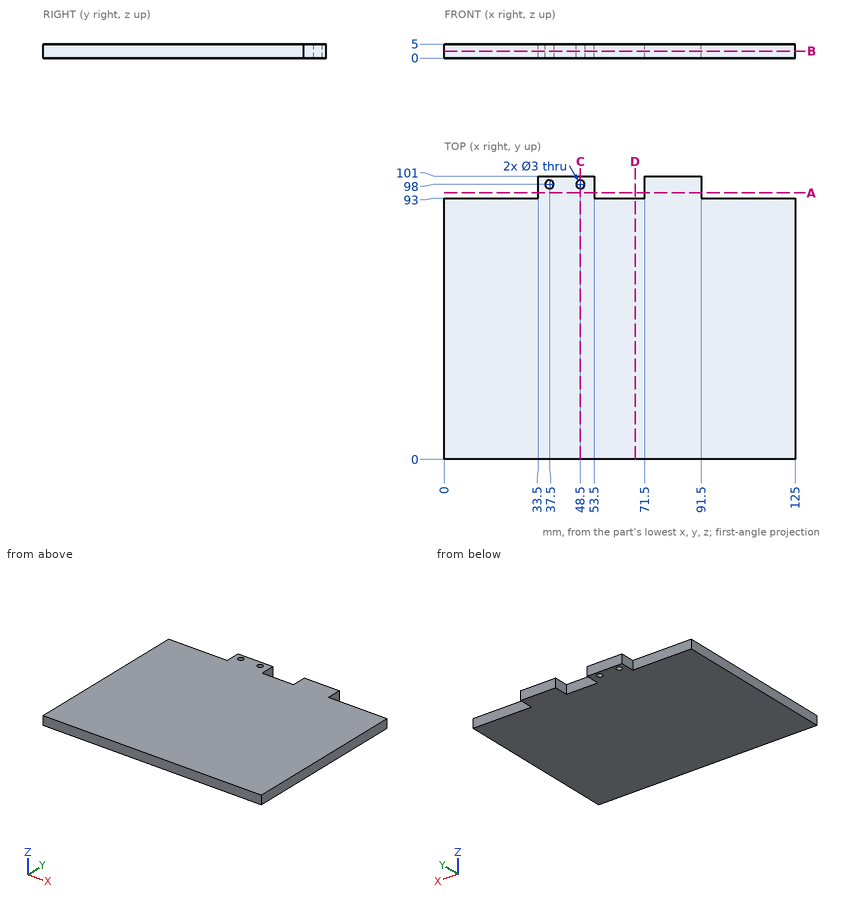
Could you check a few things on this drawing? It's one solid part, dimensions in mm from its lowest x, y, z. Give positions to 0.01 mm unless a question says otherwise; leave off trailing zeros. Order: outer loops, then holes, each group sorted by start corner. A loop starts at its lowest first (then second) coordinate and runs counter-clockwise, first axis right, second up. Notation, with made-up numbers: (49, -29) - (74, -29) arc R18 ccw to (74, 5) - close; hole circle Ø11 at (-20, 72). An arc over 180 degrees is marked (long way). One line per item, written item: value. Start each with the question number.
1. If I drill on probe 1 along X at (y, z) = (98, 1.7); probe 2 along Y at (x, z) = (48.5, 3.15); probe 3 along Y at (x, z) = (96, 4.6), over which ranges is the centre line in solid material (lowest first)?
2. Imagine slicing it at C-C on x = 48.5. List the corners of the cut face in (y, z) for me.
3. Imagine slicing it at B-B on z = 2.45. List the corners of the cut face in (x, y) for me.
4. Imagine slicing it at D-D on x = 68. List the corners of the cut face in (y, z) for me.
5. Imagine slicing it at A-A on y = 95. List the corners of the cut face in (x, z) for me.
6. For P1, Ø2.5, axis at y = 97.5, z = 2, coming from the -X side; P2, Ø2.5, axis at x = 63.5, z = 1.5, coming from the +Y side; P3, Ø2.5, axis at x = 37.5, y = 98, coming from the +Z side; P4, Ø2.5, axis at y = 98, z = 3, coming from the +X side, each with a flat end and sliding along its axis, tell me the tip position at first contact or that it passes through.
Values:
1. probe 1: 33.5 to 36, 39 to 47, 50 to 53.5, 71.5 to 91.5
1. probe 2: 0 to 96.5, 99.5 to 101
1. probe 3: 0 to 93
2. outline: (0, 0) - (96.5, 0) - (96.5, 5) - (0, 5) - close; (99.5, 0) - (101, 0) - (101, 5) - (99.5, 5) - close
3. outline: (0, 0) - (125, 0) - (125, 93) - (91.5, 93) - (91.5, 101) - (71.5, 101) - (71.5, 93) - (53.5, 93) - (53.5, 101) - (33.5, 101) - (33.5, 93) - (0, 93) - close; hole circle Ø3 at (37.5, 98); hole circle Ø3 at (48.5, 98)
4. outline: (0, 0) - (93, 0) - (93, 5) - (0, 5) - close
5. outline: (33.5, 0) - (53.5, 0) - (53.5, 5) - (33.5, 5) - close; (71.5, 0) - (91.5, 0) - (91.5, 5) - (71.5, 5) - close
6. P1: x = 33.5
6. P2: y = 93
6. P3: through
6. P4: x = 91.5
